from build123d import *

# Parameters (mm, degrees)
BOSS_EXTRUDE1_DEPTH = 25
BOSS_EXTRUDE2_START = -3
BOSS_EXTRUDE2_DEPTH = 3
CUT_EXTRUDE1_REACH  = 130.261
SKETCH3_W           = 20
SKETCH3_H           = 25
BOSS_EXTRUDE3_DEPTH = 28


with BuildPart() as part:
    # Sketch1 → Boss-Extrude1 (new body)
    with BuildSketch(Plane.XY):
        with BuildLine():
            Line((0, 0), (0, 97.6))
            ThreePointArc((0, 97.6), (0.702943725, 99.297056275), (2.4, 100))
            Line((2.4, 100), (5.6, 100))
            ThreePointArc((5.6, 100), (7.297056275, 99.297056275), (8, 97.6))
            Line((8, 97.6), (8, 0))
            Line((8, 0), (28, 0))
            Line((28, 0), (28, 115))
            Line((28, 115), (18, 115))
            Line((18, 115), (-10, 115))
            Line((-10, 115), (-23, 115))
            Line((-23, 115), (-23, 0))
            Line((-23, 0), (0, 0))
        make_face()
        with BuildLine():
            Line((18, 108.6), (18, 10))
            Line((18, 10), (20, 10))
            Line((20, 10), (20, 108.6))
            ThreePointArc((20, 108.6), (20.702943725, 110.297056275), (22.4, 111))
            Line((22.4, 111), (22.6, 111))
            ThreePointArc((22.6, 111), (24.297056275, 110.297056275), (25, 108.6))
            Line((25, 108.6), (25, 5.4))
            ThreePointArc((25, 5.4), (24.297056275, 3.702943725), (22.6, 3))
            Line((22.6, 3), (13.4, 3))
            ThreePointArc((13.4, 3), (11.702943725, 3.702943725), (11, 5.4))
            Line((11, 5.4), (11, 104))
            Line((11, 104), (-3, 104))
            Line((-3, 104), (-3, 5.4))
            ThreePointArc((-3, 5.4), (-3.702943725, 3.702943725), (-5.4, 3))
            Line((-5.4, 3), (-17.6, 3))
            ThreePointArc((-17.6, 3), (-19.297056275, 3.702943725), (-20, 5.4))
            Line((-20, 5.4), (-20, 108.6))
            ThreePointArc((-20, 108.6), (-19.297056275, 110.297056275), (-17.6, 111))
            Line((-17.6, 111), (-15.4, 111))
            ThreePointArc((-15.4, 111), (-13.702943725, 110.297056275), (-13, 108.6))
            Line((-13, 108.6), (-13, 12))
            Line((-13, 12), (-11, 12))
            Line((-11, 12), (-11, 108.6))
            ThreePointArc((-11, 108.6), (-10.297056275, 110.297056275), (-8.6, 111))
            Line((-8.6, 111), (15.6, 111))
            ThreePointArc((15.6, 111), (17.297056275, 110.297056275), (18, 108.6))
        make_face(mode=Mode.SUBTRACT)
    extrude(amount=BOSS_EXTRUDE1_DEPTH)

    # Sketch2 → Boss-Extrude2 (add)
    with BuildSketch(Plane.XY.offset(BOSS_EXTRUDE2_START)):
        with BuildLine():
            Line((28, 115), (-23, 115))
            Line((-23, 115), (-23, 0))
            Line((-23, 0), (0, 0))
            Line((0, 0), (0, 97.6))
            ThreePointArc((0, 97.6), (0.702943725, 99.297056275), (2.4, 100))
            Line((2.4, 100), (5.6, 100))
            ThreePointArc((5.6, 100), (7.297056275, 99.297056275), (8, 97.6))
            Line((8, 97.6), (8, 0))
            Line((8, 0), (28, 0))
            Line((28, 0), (28, 115))
        make_face()
    extrude(amount=BOSS_EXTRUDE2_DEPTH)

    # Sketch3 → Cut-Extrude1 (cut, up to next)
    with BuildSketch(Plane(origin=(28, 0, 0), x_dir=(0, 0, -1), z_dir=(1, 0, 0)), mode=Mode.PRIVATE) as cut_extrude1_sk1:
        with Locations((-11, 82.5)):
            Rectangle(SKETCH3_W, SKETCH3_H)
    cut_extrude1_tool1 = extrude(cut_extrude1_sk1.sketch, amount=-CUT_EXTRUDE1_REACH, mode=Mode.PRIVATE) & part.part
    add(cut_extrude1_tool1.solids().sort_by_distance((28, 82.5, 11))[0], mode=Mode.SUBTRACT)

    # Sketch4 → Boss-Extrude3 (add)
    with BuildSketch(Plane(origin=(0, 0, -3), x_dir=(-1, 0, 0), z_dir=(0, 0, -1))):
        Polygon((-28, 99), (-31, 99), (-31, 96.6), (-34, 96.6), (-34, 100.6), (-28, 104), align=None)
        Polygon((-28, 61), (-28, 66), (-31, 66), (-31, 68.4), (-34, 68.4), (-34, 64.4), align=None)
    extrude(amount=-BOSS_EXTRUDE3_DEPTH)


solid = part.part
Work out the finished part from the listing and answer in its coordinate system (mm). A direction names the side the tool comes from. Coordinates: 2 decimals unless noted, no trailing zeros. Order: outer loops, then holes, each group sorted by start corner. A loop starts at its lowest first (then second) coordinate and runs counter-clockwise, first axis right, second up. Notation, with made-up numbers: (20.25, 4.25) - (67.25, 4.25) arc R22 ccw to (67.25, 23.25) - close; hole circle Ø3 at (-27, -4). An arc over 180 degrees is marked (long way). Put each result on its own line as item: value. Start each with the question number.
1) Find the intervals of material crossed by line 1 (X direction, y = 94.5, z = 13.75); line 2 (X direction, y = 56.5, z = 20); line 3 (X direction, y = 5.5, z = 3.5), in increasing order. Write a range as from..to.
2) For a pull along Y with two mould halves and no side action, classify faces 1 (the flat face through (-11, 3, 12)), 2 (the flat face through (31, 102.3, 10.8)), 3 (the cylindrical face through (0.684, 99.278, 10.804)), 4 (the flat face through (28, 30, 11)) as released by +Y, released by -Y, zero draft, split by the parting line, or undercut.
3) Find section A-A (y = 18). Give the vertices of the cut face in (x, z), plus the area to 3 significant figures.
4) For faces 5 (the flat face through (-20, 56, 12)), 6 (the flat face through (27, 95, 11)), 7 (the flat face through (32, 96.6, 11)), 8 (the flat face through (31, 62.7, 10.8)), 9 (the flat face through (31, 67, 11)), determine the directions among +Z, -Z, +X, -X, +Y, -Y from which every point of the face is accessible in a straight line to the end or side of a thin tool.
5) Find section B-B (y = 84). Give the vertices of the cut face in (x, z).
6) Find section C-C (x = 9.5). Give the vertices of the cut face in (y, z), plus the area to 4 significant figures.
7) Flat-ended cylindrical pins translate along their axes: pin 1 (3 mm diameter, centred on y = 78, z = 12, fed in from +X); pin 2 (0.9 mm diameter, centred on x = 32.5, z = 8, fed in from -Y) (3 decimals); pin 3 (1.5 mm diameter, centred on x = 29.5, z = 14.5, fed in from +Y) (3 decimals). Find the tip coordinate at first contact, or state that the pin passes through.
Results list:
1. line 1: x = -23..-20, -13..-11, -3..0, 8..11, 18..20
1. line 2: x = -23..-20, -13..-11, -3..0, 8..11, 18..20, 25..28
1. line 3: x = -23..-20, -3..0, 8..11, 25..28
2. face 1: undercut
2. face 2: released by +Y
2. face 3: released by -Y
2. face 4: zero draft
3. outline: (-23, -3) - (0, -3) - (0, 25) - (-3, 25) - (-3, 0) - (-11, 0) - (-11, 25) - (-13, 25) - (-13, 0) - (-20, 0) - (-20, 25) - (-23, 25) - close; (8, -3) - (28, -3) - (28, 25) - (25, 25) - (25, 0) - (20, 0) - (20, 25) - (18, 25) - (18, 0) - (11, 0) - (11, 25) - (8, 25) - close
3. area: 529 mm^2
4. face 5: +Z
4. face 6: +X
4. face 7: +Z, -Z, +X
4. face 8: +Z, -Z, +X, -Y
4. face 9: +Z, -Z
5. outline: (-23, -3) - (0, -3) - (0, 25) - (-3, 25) - (-3, 0) - (-11, 0) - (-11, 25) - (-13, 25) - (-13, 0) - (-20, 0) - (-20, 25) - (-23, 25) - close; (8, -3) - (28, -3) - (28, 1) - (25, 1) - (25, 0) - (20, 0) - (20, 25) - (18, 25) - (18, 0) - (11, 0) - (11, 25) - (8, 25) - close; (25, 21) - (28, 21) - (28, 25) - (25, 25) - close
6. outline: (0, -3) - (115, -3) - (115, 25) - (111, 25) - (111, 0) - (104, 0) - (104, 25) - (0, 25) - close
6. area: 3,045 mm^2
7. pin 1: stops at x = 20
7. pin 2: stops at y = 63.295
7. pin 3: stops at y = 103.575
